```python
from build123d import *

# Parameters (mm, degrees)
BOSS_EXTRUDE1_DEPTH = 52
BOSS_EXTRUDE2_START = -34
BOSS_EXTRUDE2_DEPTH = 34
SKETCH2_3_R         = 9
CUT_EXTRUDE2_DEPTH  = 144.697599145
FILLET1_R           = 15
RIB3_REACH          = 140.456
SKETCH4_WALL_W      = 410.665096048
SKETCH4_WALL_H      = 15


with BuildPart() as part:
    # Sketch1 → Boss-Extrude1 (new body)
    with BuildSketch(Plane.XY):
        with BuildLine():
            Line((-54, 34), (54, 34))
            ThreePointArc((54, 34), (88, 0), (54, -34))
            Line((54, -34), (-54, -34))
            ThreePointArc((-54, -34), (-88, 0), (-54, 34))
        make_face()
        with BuildLine():
            Line((-54, 15), (54, 15))
            ThreePointArc((54, 15), (69, 0), (54, -15))
            Line((54, -15), (-54, -15))
            ThreePointArc((-54, -15), (-69, 0), (-54, 15))
        make_face(mode=Mode.SUBTRACT)
    extrude(amount=BOSS_EXTRUDE1_DEPTH)

    # Sketch2 → Boss-Extrude2 (add)
    with BuildSketch(Plane.XY.offset(52).offset(BOSS_EXTRUDE2_START)):
        with BuildLine():
            Line((29, 76), (29, 34))
            Line((29, 34), (54, 34))
            ThreePointArc((54, 34), (67.647767834, 31.140623519), (79, 23.043437244))
            Line((79, 23.043437244), (79, 76))
            ThreePointArc((79, 76), (54, 101), (29, 76))
        make_face()
    extrude(amount=BOSS_EXTRUDE2_DEPTH)

    # Sketch2<3> → Cut-Extrude2 (cut, through all)
    with BuildSketch(Plane.XY.offset(52)):
        with Locations((54, 76)):
            Circle(SKETCH2_3_R)
    extrude(amount=-CUT_EXTRUDE2_DEPTH, mode=Mode.SUBTRACT)

    # Fillet1
    fillet1_edges = [part.edges().sort_by_distance(p)[0] for p in [
        (29, 34, 35),
    ]]
    fillet(fillet1_edges, radius=FILLET1_R)

    # Sketch4 wall → Rib3 (add, up to next)
    with BuildSketch(Plane(origin=(-15.293433294, 63.226194681, 35), x_dir=(0.855125243419, 0.518421467599, 0), z_dir=(-0.518421467599, 0.855125243419, 0)), mode=Mode.PRIVATE) as rib3_sk1:
        Rectangle(SKETCH4_WALL_W, SKETCH4_WALL_H)
    rib3_tool1 = extrude(rib3_sk1.sketch, amount=-RIB3_REACH, mode=Mode.PRIVATE) - part.part
    add(rib3_tool1.solids().sort_by_distance((-15.293433294, 63.226194681, 35))[0])


solid = part.part
```
Work out the finished part from the listing and answer in its coordinate system (mm). A direction names the side the tool comes from. Coordinates: 2 decimals unless noted, no trailing zeros. Write each loop counter-clockwise with the first axis right and the second up, starting at its lowest first coordinate (ties: lowest second). Pieces come first, ordered by that corner, then holes. Notation, with made-up numbers: (-20, -25.75) - (9, -25.75) arc R8 ccw to (9, -19.75) - close; hole circle Ø5 at (20, 64). An arc over 180 degrees is marked (long way). Answer as a JSON object with one key per item and string values.
Q1. Find section A-A (z = 15.5). Write down the section's boundary in (x, y).
Results list:
{"outline": "(-54, -34) - (54, -34) arc R34 ccw to (54, 34) - (-54, 34) arc R34 ccw to start; hole (-54, -15) - (54, -15) arc R15 ccw to (54, 15) - (-54, 15) arc R15 ccw to start"}
Q2. Consider L1, parallel to Y at x = 54, z = 32; L2, parallel to Y at x = 27.5, z = 7; L3, parallel to Y at x = 62, z = 25. Determine where each line is inside the solid, lowest interval first. Write a range as from..to.
Results list:
{"L1": "y = -34..-15, 15..67, 85..101", "L2": "y = -34..-15, 15..34", "L3": "y = -33.05..-12.69, 12.69..71.88, 80.12..99.69"}
Q3. Find section D-D (y = 36). Write down the section's boundary in (x, z).
Results list:
{"outline": "(-60.2, 27.5) - (21.48, 27.5) - (21.48, 18) - (79, 18) - (79, 52) - (21.48, 52) - (21.48, 42.5) - (-60.2, 42.5) - close"}
Q4. For a pull along Y with two mould halves and no side action, classify faces 4 (the cylindrical face through (69, 0, 26)), 5 (the cylindrical face through (24.72, 38.51, 22.82)), 6 (the cylindrical face through (86.2, -10.92, 25.64)) as pulls with the +Y half, pulls with the -Y half, needs draft (parallel to the pull), parting line crosses it, or undercut.
Results list:
{"face 4": "undercut", "face 5": "pulls with the +Y half", "face 6": "parting line crosses it"}
Q5. Which of the six approach directions +Z, -Z, +X, -X, +Y, -Y give full straight-line access (tool end or side, diameter ignored) to faces 1 (the flat face through (29, 63, 47)), 2 (the flat face through (-1, 34, 14)), 3 (the cylindrical face through (-69, 0, 26))?
Results list:
{"face 1": "+Z, -X, +Y", "face 2": "-Z, -X, +Y", "face 3": "+Z, -Z"}
Q6. Find section B-B (y = 0). Write down the section's boundary in (x, z), plus the area to 3 significant figures.
Results list:
{"outline": "(-88, 0) - (-69, 0) - (-69, 52) - (-88, 52) - close; (69, 0) - (88, 0) - (88, 52) - (69, 52) - close", "area": "1,980 mm^2"}
Q7. Given pin 1 Ø4 at (x, z) = (3, 46) entering from +Y; pin 2 Ø5 at (y, z) = (83, 20.5) entering from -X; pin 3 Ø1.5 at (x, z) = (56.5, 44) entering from +Y; pin 4 Ø12 at (x, y) = (31, 35.5) entering from -Z, each flat-ended and moving along its own axis, determine where each tip first touches the part or whether it passes through.
Results list:
{"pin 1": "stops at y = 34", "pin 2": "stops at x = 29.41", "pin 3": "stops at y = 100.94", "pin 4": "stops at z = 0"}
Q8. Find section C-C (x = 77). Write down the section's boundary in (y, z).
Results list:
{"outline": "(-25.04, 0) - (25.04, 0) - (25.04, 18) - (85.8, 18) - (85.8, 52) - (-25.04, 52) - close"}
